Part model, mm, in its own coordinate system. A direction names the side the tool comes from. Give positions to 0.01 mm unless a question says otherwise; leave off trailing zeros. Order: outer loops, then holes, each group sorted by start corner. A loop starts at its lowest first (then second) coordinate and runs counter-clockwise, first axis right, second up. Notation, with made-up numbers: M 51,-26.5 L 92,-26.5 A4 ccw 92,-19.5 Z; hole C -22.75,24.25 d6. An arc over 180 degrees is marked long. Return JSON: item names as keys, results as strings.
from build123d import *

# Parameters (mm, degrees)
BOSS_EXTRU_1_DEPTH      = 10
ESQUISSE3_R             = 2.25
ENL_V_MAT_EXTRU_1_DEPTH = 5
ESQUISSE5_R             = 11
ENL_V_MAT_EXTRU_2_DEPTH = 10
ESQUISSE6_R             = 12.5
ENL_V_MAT_EXTRU_3_DEPTH = 1
ENL_V_START             = -1
ESQUISSE7_R             = 12.5
ENL_V_MAT_EXTRU_4_DEPTH = 1
ENL_V_MAT_EXTRU_5_DEPTH = 5
ENL_V_START_2           = -4
ENL_V_MAT_EXTRU_6_DEPTH = 4
ENL_V_MAT_EXTRU_7_DEPTH = 4


with BuildPart() as part:
    # Esquisse2 → Boss.-Extru.1 (new body)
    with BuildSketch(Plane(origin=(0, 0, 0), x_dir=(1, 0, 0), z_dir=(0, 1, 0))):
        with BuildLine():
            Line((14.087488664, 0), (27.5, 0))
            Line((27.5, 0), (27.5, 5))
            Line((27.5, 5), (14.962375299, 5))
            Line((14.962375299, 5), (14, 16))
            ThreePointArc((14, 16), (0, 30), (-14, 16))
            Line((-14, 16), (-14.962375299, 5))
            Line((-14.962375299, 5), (-27.5, 5))
            Line((-27.5, 5), (-27.5, 0))
            Line((-27.5, 0), (-14.087488664, 0))
            Line((-14.087488664, 0), (-14, 1))
            Line((-14, 1), (14, 1))
            Line((14, 1), (14.087488664, 0))
        make_face()
    extrude(amount=BOSS_EXTRU_1_DEPTH)

    # Esquisse3 → Enlèv. mat.-Extru.1 (cut)
    with BuildSketch(Plane.XY):
        with Locations((-21, 5)):
            Circle(ESQUISSE3_R)
        with Locations((21, 5)):
            Circle(ESQUISSE3_R)
        Polygon((-27.5, 3), (-24.5, 0), (-27.5, 0), align=None)
        Polygon((-27.5, 10), (-27.5, 7), (-24.5, 10), align=None)
        Polygon((27.5, 7), (24.5, 10), (27.5, 10), align=None)
        Polygon((27.5, 3), (24.5, 0), (27.5, 0), align=None)
    extrude(amount=-ENL_V_MAT_EXTRU_1_DEPTH, mode=Mode.SUBTRACT)

    # Esquisse5 → Enlèv. mat.-Extru.2 (cut)
    with BuildSketch(Plane(origin=(0, 10, 0), x_dir=(1, 0, 0), z_dir=(0, 1, 0))):
        with Locations(Location((0, 16, 0), (0, 0, 270))):
            Circle(ESQUISSE5_R)
    extrude(amount=-ENL_V_MAT_EXTRU_2_DEPTH, mode=Mode.SUBTRACT)

    # Esquisse6 → Enlèv. mat.-Extru.3 (cut)
    with BuildSketch(Plane(origin=(0, 10, 0), x_dir=(1, 0, 0), z_dir=(0, 1, 0))):
        with Locations(Location((0, 16, 0), (0, 0, 270))):
            Circle(ESQUISSE6_R)
    extrude(amount=-ENL_V_MAT_EXTRU_3_DEPTH, mode=Mode.SUBTRACT)

    # Esquisse7 → Enlèv. mat.-Extru.4 (cut)
    with BuildSketch(Plane.XZ.offset(ENL_V_START)):
        with Locations(Location((0, -16, 0), (0, 0, 90))):
            Circle(ESQUISSE7_R)
    extrude(amount=ENL_V_MAT_EXTRU_4_DEPTH, mode=Mode.SUBTRACT)

    # Esquisse8 → Enlèv. mat.-Extru.5 (cut)
    with BuildSketch(Plane(origin=(0, 9, 0), x_dir=(1, 0, 0), z_dir=(0, 1, 0))):
        with BuildLine():
            Line((11.56233108, 20.75), (9.921567416, 20.75))
            ThreePointArc((9.921567416, 20.75), (11, 16), (9.921567416, 11.25))
            Line((9.921567416, 11.25), (11.56233108, 11.25))
            ThreePointArc((11.56233108, 11.25), (12.5, 16), (11.56233108, 20.75))
        make_face()
    extrude(amount=-ENL_V_MAT_EXTRU_5_DEPTH, mode=Mode.SUBTRACT)

    # Esquisse9 → Enlèv. mat.-Extru.6 (cut)
    with BuildSketch(Plane(origin=(0, 10, 0), x_dir=(1, 0, 0), z_dir=(0, 1, 0)).offset(ENL_V_START_2)):
        with BuildLine():
            Line((14, 1), (13.116009813, 11.104054068))
            ThreePointArc((13.116009813, 11.104054068), (0, 2), (-13.116009813, 11.104054068))
            Line((-13.116009813, 11.104054068), (-14, 1))
            Line((-14, 1), (14, 1))
        make_face()
    extrude(amount=ENL_V_MAT_EXTRU_6_DEPTH, mode=Mode.SUBTRACT)

    # Esquisse10 → Enlèv. mat.-Extru.7 (cut)
    with BuildSketch(Plane.XZ):
        with BuildLine():
            Line((13.116009813, -11.104054068), (14, -1))
            Line((14, -1), (-14, -1))
            Line((-14, -1), (-13.116009813, -11.104054068))
            ThreePointArc((-13.116009813, -11.104054068), (0, -2), (13.116009813, -11.104054068))
        make_face()
    extrude(amount=-ENL_V_MAT_EXTRU_7_DEPTH, mode=Mode.SUBTRACT)


solid = part.part
Q1. 3-axis set-ups, long thin cutter, end or side, ignore diameter. For faces 1 (the flat face through (11, 7, -11.25)), 2 (the flat face through (10, 1, -11)), 3 (the flat face through (18.5, 4.9, -5)), 4 (the flat face through (-0.2, 6, -1.6)): which of +Z, -Z, +X, -X, +Y, -Y reach the whole face in a straight line?
Established:
{"face 1": "+Y", "face 2": "-Y", "face 3": "-Z, +X, +Y, -Y", "face 4": "+Z, +Y"}
Q2. Band-saw the part on A-A (y = 5). Give the cut face in (x, z), then the cut area to 3 significant figures.
Established:
{"outline": "M -27.5,-5 L -23.25,-5 L -23.25,0 L -27.5,0 Z; M -18.75,-5 L -14.96,-5 L -14,-16 A14 ccw 14,-16 L 14.96,-5 L 18.75,-5 L 18.75,0 L 14.09,0 L 14,-1 L -14,-1 L -14.09,0 L -18.75,0 Z; M 23.25,-5 L 27.5,-5 L 27.5,0 L 23.25,0 Z; hole M 9.92,-20.75 L 11.56,-20.75 A12.5 ccw 11.56,-11.25 L 9.92,-11.25 A11 ccw long Z", "area": "434 mm²"}
Q3. Two-plate mould, pull along Z, no slides. Class faces 5 (the flat face through (26, 1.5, -2.5)), 6 (the cylindrical face through (0, 5, -30)), 7 (the flat face through (11.5, 4, -16.1)): +Z half, -Z half, draft (parallel to the pull), parting line (faces both ways), or undercut.
Established:
{"face 5": "draft", "face 6": "-Z half", "face 7": "undercut"}
Q4. Pin check, flat tips, straight feed: pin 1 (0.6 mm diameter, centred on x = 3.5, y = 5.5, fed in from +Z); pin 2 (5 mm diameter, centred on x = 4.5, z = -7.5, fed in from -Y); pin 3 (5 mm diameter, centred on x = -9, z = -23, fed in from +Y); pin 4 (1.8 mm diameter, centred on x = 11, y = 7, fed in from +Z). Stop position of each tip, or through.
Established:
{"pin 1": "stops at z = -1", "pin 2": "stops at y = 1", "pin 3": "stops at y = 10", "pin 4": "stops at z = -6.31"}
Q5. Band-saw the part on C-C (z = -26). Give the cut face in (x, y).
Established:
{"outline": "M -9.8,0 L -7.5,0 L -7.5,1 L -4.58,1 L -4.58,9 L -7.5,9 L -7.5,10 L -9.8,10 Z; M 4.58,1 L 7.5,1 L 7.5,0 L 9.8,0 L 9.8,10 L 7.5,10 L 7.5,9 L 4.58,9 Z"}
Q6. Probe line 1 along Z through (x, y) = (0, 9.65); line 2 along X through (y, z) = (9.3, -16); line 3 along X through (y, z) = (5.5, -4.75). List the from-to ranges inside material, lowest first.
Established:
{"line 1": "z = -30 to -28.5, -3.5 to -2", "line 2": "x = -14 to -12.5, 12.5 to 14", "line 3": "x = -27.5 to -23.19, -18.81 to 18.81, 23.19 to 27.5"}
Q7. Band-saw the part on B-B (x = -21). Give the cut face in (y, z).
Established:
{"outline": "M 0,-5 L 2.75,-5 L 2.75,0 L 0,0 Z; M 7.25,-5 L 10,-5 L 10,0 L 7.25,0 Z"}
Q8. Band-saw the part on D-D (x = 0). Give the cut face in (y, z), then the cut area to 3 significant figures.
Established:
{"outline": "M 0,-30 L 10,-30 L 10,-28.5 L 9,-28.5 L 9,-27 L 1,-27 L 1,-28.5 L 0,-28.5 Z; M 0,-3.5 L 1,-3.5 L 1,-5 L 9,-5 L 9,-3.5 L 10,-3.5 L 10,-2 L 6,-2 L 6,-1 L 4,-1 L 4,-2 L 0,-2 Z", "area": "56.0 mm²"}
